Solid Edge part; units mm, degrees
sketch "Sketch1" plane through (0, 0, 0) normal (0, 0, 1) x (1, 0, 0)
  line L0 (-37, -45) -> (37, -45)
  line L1 (37, -45) -> (37, 45)
  line L2 (37, 45) -> (-37, 45)
  line L3 (-37, 45) -> (-37, -45)
  dimension "D1" = 37
  dimension "D2" = 37
extrude "Protrusion1" add sketch "Sketch1" along normal blind 2
sketch "Sketch2" plane through (0, 0, 2) normal (0, 0, 1) x (1, 0, 0)
  line L0 (-35, -43) -> (-35, 45)
  line L1 (-35, 45) -> (-37, 45)
  line L2 (-37, 45) -> (-37, -45)
  line L3 (37, -45) -> (-37, -45)
  line L4 (37, -45) -> (37, 45)
  line L5 (37, 45) -> (35, 45)
  line L6 (35, 45) -> (35, -43)
  line L7 (35, -43) -> (-35, -43)
extrude "ExtrudedProtrusion_2" add sketch "Sketch2" along normal blind 3
sketch "Sketch3" plane through (35, 1, 3.5) normal (-1, 0, 0) x (0, -1, 0)
  line L0 (44, 1.5) -> (-33, 1.5)
  line L1 (-33, 1.5) -> (-33, 0)
  line L2 (-33, 0) -> (44, 0)
  line L3 (44, 0) -> (44, 1.5)
extrude "ExtrudedProtrusion_3" add sketch "Sketch3" along normal blind 4
sketch "Sketch4" plane through (-35, 1, 3.5) normal (1, 0, 0) x (0, 1, 0)
  line L0 (-44, 1.5) -> (33, 1.5)
  line L1 (33, 1.5) -> (33, 0)
  line L2 (33, 0) -> (-44, 0)
  line L3 (-44, 0) -> (-44, 1.5)
extrude "ExtrudedProtrusion_4" add sketch "Sketch4" along normal blind 4
sketch "Sketch5" plane through (35, 1, 3.5) normal (-1, 0, 0) x (0, -1, 0)
  spline S0 degree 3 poles (-33, -1.5) (-34.865, -1.4464) (-37.9174, -1.5297) (-41.2071, 1.135) (-43.2352, 1.3829) (-44, 1.5) knots 0 0 0 0 0.440598 0.817285 1 1 1 1
  line L0 (-44, -1.5) -> (-33, -1.5)
  line L1 (-44, 1.5) -> (-44, -1.5)
extrude "ExtrudedProtrusion_5" add sketch "Sketch5" along normal blind 70
fillet "Round_5" radius 1 2 edges at (33, 34, 3.5) (-33, 34, 3.5)
sketch "Sketch6" plane through (0, 45, 2.5) normal (0, 1, 0) x (-1, 0, 0)
  line L0 (37, -2.5) -> (-37, -2.5)
  line L1 (-37, -2.5) -> (-37, 2.5)
  line L2 (-37, 2.5) -> (37, 2.5)
  line L3 (37, 2.5) -> (37, -2.5)
extrude "ExtrudedProtrusion_6" add sketch "Sketch6" along normal blind 2
sketch "Sketch7" plane through (0, -4.5, 2) normal (0, 0, 1) x (1, 0, 0)
  line L0 (12.5, -30.5) -> (-12.5, -30.5)
  line L1 (-12.5, -30.5) -> (-12.5, -38.5)
  line L2 (-12.5, -38.5) -> (12.5, -38.5)
  line L3 (12.5, -38.5) -> (12.5, -30.5)
  dimension "D1" = 12.5
  dimension "D2" = 12.5
extrude "ExtrudedCutout_1" cut sketch "Sketch7" against normal blind 2
sketch "Sketch8" plane through (0, -43, 2.5) normal (0, 1, 0) x (1, 0, 0)
  line L0 (-31, -1) -> (31, -1)
  line L1 (31, -1) -> (31, -2.5)
  line L2 (31, -2.5) -> (-31, -2.5)
  line L3 (-31, -2.5) -> (-31, -1)
extrude "ExtrudedProtrusion_7" add sketch "Sketch8" along normal blind 4
sketch "Sketch9" plane through (0, 0, 0) normal (1, 0, 0) x (0, 1, 0)
  line L0 (47, 0) -> (-28, 0)
  line L1 (-28, 0) -> (-28, 5)
  line L2 (-28, 5) -> (47, 5)
  line L3 (47, 5) -> (47, 0)
extrude "ExtrudedCutout_2" cut sketch "Sketch9" along normal mid plane 75
The model under review builds one solid part; all positions refer to its coordinate system, in mm. A direction names the side the tool comes from. Give positions to 0.01 mm unless a question says otherwise; leave off trailing zeros. Order: outer loops, then holes, each group sorted by start corner. A loop starts at its lowest first (then second) coordinate and runs counter-clockwise, first axis right, second up. Notation, with made-up numbers: (61.5, 13.25) -> (116.5, 13.25) arc R18 ccw to (116.5, 42.25) -> close; hole circle Ø10 at (69, -24.75). An arc over 180 degrees is marked (long way). Write item = value, one per line. Start each with the question number.
(1) Take a section at A-A (x = 6.5). Write out the cut boundary in (y, z), plus the area to 3 significant figures.
(2) Take a section at C-C (y = -40.5). Write out the cut boundary in (x, z).
(3) Take a section at D-D (x = 27.5). Write out the cut boundary in (y, z), plus the area to 3 significant figures.
(4) Draft analysis for pull direction Z (two halves, no side actions). For faces 1 (the flat face through (0, -43, 2)), 2 (the flat face through (37, -37, 2)), 3 (the flat face through (-1, -40, 5)), state which applies: +Z half, -Z half, draft (parallel to the pull), parting line (faces both ways), or undercut.
(5) For L1, parallel to X at y = -29.25, z = 4.05; L2, parallel to X at y = -37.25, z = 1; L3, parallel to Z at x = 32.5, y = -42.5, list the stretches that pass through material, from the lowest coordinate up. Write a range as from..to.
(6) Tool access review of faces 4 (the flat face through (0, -35, 1)), 5 (the flat face through (0, -34, 2)), 6 (the flat face through (-12.5, -39, 1)), 7 (the flat face through (0, -39, 4)): name each direction out of +Z, -Z, +X, -X, +Y, -Y from which nothing blocks a thin tool from reaching the whole face with its end or side.
(7) For pin 1 Ø1 at (x, y) = (-27.5, -30.5) entering from +Z; pin 2 Ø1.5 at (x, z) = (-1, 3.5) entering from +Y, all flat-tipped, find the tip position at first contact; note any pin that passes through.
(8) Take a section at B-B (y = -36.25). Write out the cut boundary in (x, z).
Returned:
q1.outline = (-45, 0) -> (-43, 0) -> (-43, 3.5) -> (-39, 3.5) -> (-39, 5) -> (-45, 5) -> close; (-35, 0) -> (-28, 0) -> (-28, 2) -> (-35, 2) -> close
q1.area = 30.0 mm²
q2.outline = (-37, 0) -> (-12.5, 0) -> (-12.5, 2) -> (-35, 2) -> (-35, 3.5) -> (35, 3.5) -> (35, 2) -> (12.5, 2) -> (12.5, 0) -> (37, 0) -> (37, 5) -> (-37, 5) -> close
q3.outline = (-45, 0) -> (-28, 0) -> (-28, 2) -> (-43, 2) -> (-43, 3.5) -> (-39, 3.5) -> (-39, 5) -> (-45, 5) -> close
q3.area = 46.0 mm²
q4.face_1 = undercut
q4.face_2 = draft
q4.face_3 = +Z half
q5.L1 = -37..-31, 31..37
q5.L2 = -37..-12.5, 12.5..37
q5.L3 = 0..2, 3.5..5
q6.face_4 = +Z, -Z
q6.face_5 = +Y
q6.face_6 = -Z
q6.face_7 = +Z, +Y
q7.pin_1 = 2
q7.pin_2 = -39
q8.outline = (-37, 0) -> (-12.5, 0) -> (-12.5, 2) -> (-35, 2) -> (-35, 3.5) -> (-31, 3.5) -> (-31, 5) -> (-37, 5) -> close; (12.5, 0) -> (37, 0) -> (37, 5) -> (31, 5) -> (31, 3.5) -> (35, 3.5) -> (35, 2) -> (12.5, 2) -> close
